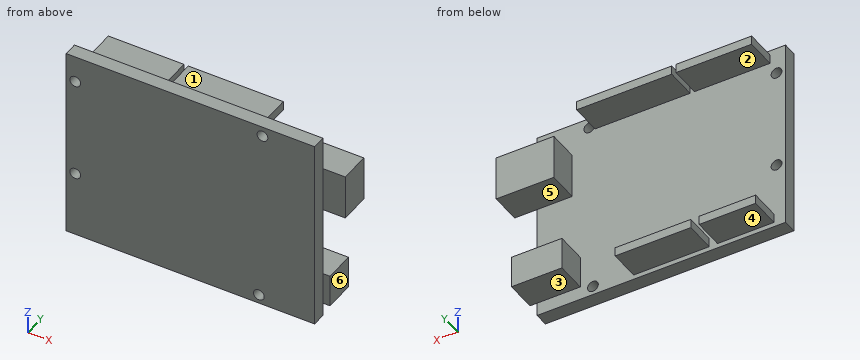
```python
from build123d import *

# Parameters (mm, degrees)
SKETCH1_W           = 69
SKETCH1_H           = 54
SKETCH1_R           = 1.5
BOSS_EXTRUDE1_DEPTH = 3.8
SKETCH2_W           = 16
SKETCH2_H           = 12.5
SKETCH2_W_2         = 14
SKETCH2_H_2         = 9
SKETCH2_W_3         = 21
SKETCH2_H_3         = 2.5
SKETCH2_W_4         = 26.4
SKETCH2_W_5         = 15.7
BOSS_EXTRUDE2_DEPTH = 8.5


with BuildPart() as part:
    # Sketch1 → Boss-Extrude1 (new body)
    with BuildSketch(Plane(origin=(0, 0, 0), x_dir=(1, 0, 0), z_dir=(0, 1, 0))):
        with Locations((0, 27)):
            Rectangle(SKETCH1_W, SKETCH1_H)
        with Locations((-32, 7.5)):
            Circle(SKETCH1_R, mode=Mode.SUBTRACT)
        with Locations((-32, 35.5)):
            Circle(SKETCH1_R, mode=Mode.SUBTRACT)
        with Locations((19, 51.5)):
            Circle(SKETCH1_R, mode=Mode.SUBTRACT)
        with Locations((20, 2.75)):
            Circle(SKETCH1_R, mode=Mode.SUBTRACT)
    extrude(amount=BOSS_EXTRUDE1_DEPTH)

    # Sketch2 → Boss-Extrude2 (add)
    with BuildSketch(Plane(origin=(0, 3.8, 0), x_dir=(1, 0, 0), z_dir=(0, 1, 0))):
        with Locations((32.75, 15.5)):
            Rectangle(SKETCH2_W, SKETCH2_H)
        with Locations((29.5, 45.75)):
            Rectangle(SKETCH2_W_2, SKETCH2_H_2)
        with Locations((-19.7, 2.55)):
            Rectangle(SKETCH2_W_3, SKETCH2_H_3)
        with Locations((5.2, 2.55)):
            Rectangle(SKETCH2_W_4, SKETCH2_H_3)
        with Locations((-23.45, 51.45)):
            Rectangle(SKETCH2_W_5, SKETCH2_H_3)
        with Locations((-2.8, 51.45)):
            Rectangle(SKETCH2_W_3, SKETCH2_H_3)
    extrude(amount=BOSS_EXTRUDE2_DEPTH)


solid = part.part
```
Could you check a few things on this model? Use its own coordinates, in mm. Face numbers are marked on the shaded views. A direction names the side the tool comes from. Round coordinates to 2 decimals unless told otherwise and drop trailing zeros. Loops run counter-clockwise (first coordinate to the right, second up) from the corner with the lowest first, then second, coordinate; pieces in that order, holes last. Notation, with made-up numbers: M 87.5,-39 L 99.5,-39 A28 ccw 99.5,-6 Z; hole C 69,-4 d7. An arc over 180 degrees is marked long. Put each result on its own line as item: value.
Q1. Imagine slicing it at B-B (y = 2.5). Write out the boundary of the cut face in (x, z).
Check result:
outline: M -34.5,-54 L 34.5,-54 L 34.5,0 L -34.5,0 Z; hole C -32,-35.5 d3; hole C -32,-7.5 d3; hole C 19,-51.5 d3; hole C 20,-2.75 d3
Q2. For pin 1 (4 mm diameter, centred on y = 1.5, z = -38.5, fed in from +X); pin 2 (12 mm diameter, centred on x = 1, z = -23, fed in from +Y); pin 3 (3 mm diameter, centred on x = -24.5, y = 6, fed in from -Z), each with a flat end and sliding along its axis, tell me the tip position at first contact or that it passes through.
Check result:
pin 1: x = 34.5
pin 2: y = 3.8
pin 3: z = -52.7
Q3. On a 3-axis mill with a long thin cutter (end or side, diameter ignored), from which of +Z, -Z, +X, -X, +Y, -Y can I reach the whole of each face in a straight line? I mean the marked faces 4, 5 and 6. Say none if no direction works.
Check result:
face 4: -Z, +X, -X, +Y
face 5: +X, -X, +Y
face 6: -Z, +X, +Y, -Y
Q4. Imagine slicing it at C-C (x = -17.5). Write out the boundary of the cut face in (y, z).
Check result:
outline: M 0,-54 L 3.8,-54 L 3.8,-52.7 L 12.3,-52.7 L 12.3,-50.2 L 3.8,-50.2 L 3.8,-3.8 L 12.3,-3.8 L 12.3,-1.3 L 3.8,-1.3 L 3.8,0 L 0,0 Z
Q5. Imagine slicing it at A-A (z = -2.75). Write out the boundary of the cut face in (x, y).
Check result:
outline: M -34.5,0 L 18.5,0 L 18.5,3.8 L 18.4,3.8 L 18.4,12.3 L -8,12.3 L -8,3.8 L -9.2,3.8 L -9.2,12.3 L -30.2,12.3 L -30.2,3.8 L -34.5,3.8 Z; M 21.5,0 L 34.5,0 L 34.5,3.8 L 21.5,3.8 Z
Q6. Thinking about a two-plate mould opening in Z: for the marked faces 1, 2 and 3, which applies, released by +Z, released by -Z, zero draft, split by the parting line, or undercut?
Check result:
face 1: released by +Z
face 2: undercut
face 3: released by -Z
Q7. I need wall thicknesses on probe 1 along Z at (x, y) = (-32, 2.25); probe 2 along X at (y, z) = (0.85, -7.5); probe 3 along X at (y, z) = (1.4, -2.75). Which ranges of each line are inside material? Lowest first, please.
Check result:
probe 1: -54 to -37, -34 to -9, -6 to 0
probe 2: -34.5 to -33.5, -30.5 to 34.5
probe 3: -34.5 to 18.5, 21.5 to 34.5
Q8. Imagine slicing it at D-D (z = -20). Write out the boundary of the cut face in (x, y), then the cut area to 3 significant figures.
Check result:
outline: M -34.5,0 L 34.5,0 L 34.5,3.8 L 40.75,3.8 L 40.75,12.3 L 24.75,12.3 L 24.75,3.8 L -34.5,3.8 Z
area: 398 mm2
